Source: CAD feature listing. Evaluate the final solid. Frame: model axes, mm. Give positions to 0.01 mm unless a question says otherwise; leave off trailing zeros. Order: outer loops, then holes, each group sorted by start corner. A loop starts at its lowest first (then second) coordinate and runs counter-clockwise, first axis right, second up. Notation, with made-up numbers: M -26,-4.5 L 30,-4.5 A27 ccw 30,27.5 Z; hole C 88,72 d2. An arc over 180 degrees is marked long. Use CSV: the item, a comma, the result in double quotes. Start each with the question number.
1. Section query A-A, the plane z = 9.75. Return the cut outline in (x, y), plus the area to 3 significant figures.
2. Line query: line 1 along Z through (x, y) = (-4.75, 10.75); line 2 along Y through (x, z) = (0.25, 19); line 3 along X through (y, z) = (7, 8.75). Output: solid intervals per line, ascending. Write a range as [from, to].
3. Pin query (flat end, axial travel): P1, Ø1, axis at y = 7.5, z = 4.5, coming from the -X side; P2, Ø4, axis at y = -8, z = 4.5, coming from the +X side; P3, Ø1, axis at y = 2, z = 19, coming from the -X side; P4, Ø8, axis at x = 8, y = -8, coming from the -Z side. Return the tip coordinate at first contact, or that it passes through.
Autodesk Inventor part; units mm, degrees
ref_plane "YZ Plane" through (0, 0, 0) normal (1, 0, 0) x (0, 1, 0)
ref_plane "XZ Plane" through (0, 0, 0) normal (0, 1, 0) x (-1, 0, 0)
ref_plane "XY Plane" through (0, 0, 0) normal (0, 0, 1) x (1, 0, 0)
sketch "Sketch1" plane through (0, 0, 0) normal (0, 0, 1) x (1, 0, 0)
  circle A0 centre (0, 0) radius 12.25
  dimension "d0" = 24.5
extrude "Extrusion1" add sketch "Sketch1" along normal blind 26
chamfer "Chamfer1" distance 0.5 angle 45 1 edges at (-12.25, 0, 0)
chamfer "Chamfer2" distance 0.5 angle 45 1 edges at (-12.25, 0, 26)
properties part number "gearbox"
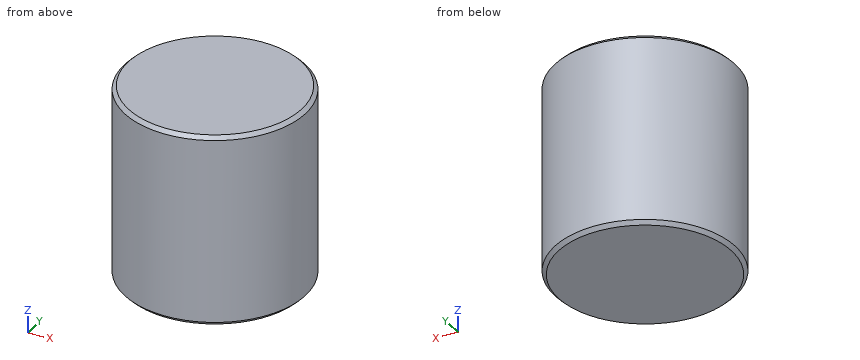
Result set:
1,outline,"C 0,0 d24.5"
1,area,"471 mm2"
2,line 1,"[0, 26]"
2,line 2,"[-12.25, 12.25]"
2,line 3,"[-10.05, 10.05]"
3,P1,"x = -10.05"
3,P2,"x = 10.68"
3,P3,"x = -12.16"
3,P4,"z = 0"
